Model file for the job. Use its own axes, mm. Coordinates: 2 decimals unless noted, no trailing zeros. Loops run counter-clockwise (first coordinate to the right, second up) from the corner with the lowest first, then second, coordinate; pieces in that order, holes last.
from build123d import *

# Parameters (mm, degrees)
SKETCH1_R           = 7.62
BOSS_EXTRUDE1_DEPTH = 609.6
FILLET1_R           = 0.25
SKETCH2_W           = 1.27
SKETCH2_H           = 91.44
SKETCH4_W           = 2.6416
SKETCH4_H           = 1.397


with BuildPart() as part:
    # Sketch1 → Boss-Extrude1 (new body)
    with BuildSketch(Plane.XY):
        with Locations(Location((0, 0, 0), (0, 0, 180))):
            Circle(SKETCH1_R)
    extrude(amount=BOSS_EXTRUDE1_DEPTH)

    # Fillet1
    fillet1_edges = [part.edges().sort_by_distance(p)[0] for p in [
        (7.62, 0, 0),
        (7.62, 0, 609.6),
    ]]
    fillet(fillet1_edges, radius=FILLET1_R)

    # Sketch2 → Cut-Revolve2 (revolve, cut)
    with BuildSketch(Plane(origin=(0, 0, 0), x_dir=(1, 0, 0), z_dir=(0, 1, 0)), mode=Mode.PRIVATE) as cut_revolve2_sk:
        with Locations((6.985, -45.72)):
            Rectangle(SKETCH2_W, SKETCH2_H)
    cut_revolve2 = revolve(cut_revolve2_sk.sketch.rotate(Axis((0, 0, 0.780201326), (0, 0, 1)), 180), axis=Axis((0, 0, 0.780201326), (0, 0, 1)), mode=Mode.SUBTRACT)

    # Sketch4 → Cut-Revolve3 (revolve, cut)
    with BuildSketch(Plane(origin=(0, 0, 0), x_dir=(1, 0, 0), z_dir=(0, 1, 0)), mode=Mode.PRIVATE) as cut_revolve3_sk:
        with Locations((6.35, -38.7985)):
            Rectangle(SKETCH4_W, SKETCH4_H)
    cut_revolve3 = revolve(cut_revolve3_sk.sketch.rotate(Axis((0, 0, 0), (0, 0, 1)), 180), axis=Axis((0, 0, 0), (0, 0, 1)), mode=Mode.SUBTRACT)

    # Mirror1: Cut-Revolve2, Cut-Revolve3 across plane
    add(cut_revolve2.mirror(Plane.XY.offset(304.8)), mode=Mode.SUBTRACT)
    add(cut_revolve3.mirror(Plane.XY.offset(304.8)), mode=Mode.SUBTRACT)


solid = part.part
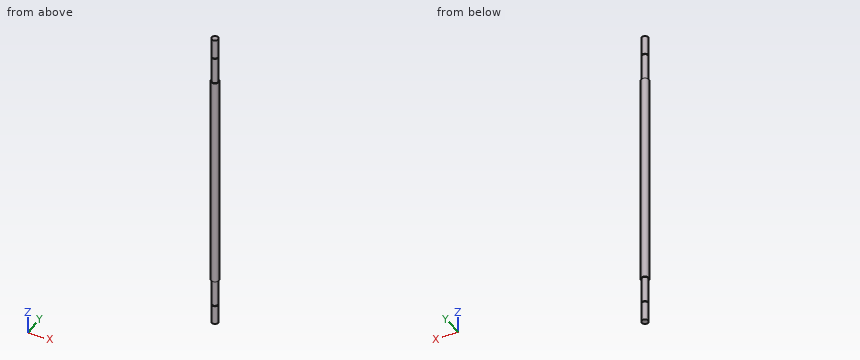
Q1. Slice it at A-A (x = 0). List the corners of the cut face in (y, z).
Answers:
outline: (-7.62, 91.44) - (-6.35, 91.44) - (-6.35, 39.5) - (-5.03, 39.5) - (-5.03, 38.1) - (-6.35, 38.1) - (-6.35, 0) - (6.35, 0) - (6.35, 38.1) - (5.03, 38.1) - (5.03, 39.5) - (6.35, 39.5) - (6.35, 91.44) - (7.62, 91.44) - (7.62, 518.16) - (6.35, 518.16) - (6.35, 570.1) - (5.03, 570.1) - (5.03, 571.5) - (6.35, 571.5) - (6.35, 609.6) - (-6.35, 609.6) - (-6.35, 571.5) - (-5.03, 571.5) - (-5.03, 570.1) - (-6.35, 570.1) - (-6.35, 518.16) - (-7.62, 518.16) - close
Q2. Slice it at C-C (z = 225). List the corners of the cut face in (x, y).
Answers:
outline: circle Ø15.24 at (0, 0)
Q3. Flat gauge pins, fed straight in: P1, Ø5, axis at x = -5.5, z = 444.5, coming from the -Y side; P2, Ø2, axis at x = 5, z = 95.5, coming from the -Y side. Where does each tip first touch, or does it go through?
Answers:
P1: stops at y = -7
P2: stops at y = -6.49
Q4. Drill centre lines: line 1 (Z direction, x = -5, y = 1); line 2 (Z direction, x = 4.5, y = -4.75); line 3 (Y direction, x = 3.75, z = 534.5). Where is each one in solid material? Low to high.
Answers:
line 1: z = 0 to 38.1, 39.5 to 570.1, 571.5 to 609.6
line 2: z = 91.44 to 518.16
line 3: y = -5.12 to 5.12
